from build123d import *

# Parameters (mm, degrees)
SKETCH_1_W          = 280
SKETCH_1_H          = 150
EXTRUDE_1_DEPTH     = 5
SKETCH_2_W          = 280
SKETCH_2_H          = 25
EXTRUDE_3_DEPTH     = 10
CUT_EXTRUDE_1_DEPTH = 500
SKETCH_7_R          = 4
CUT_EXTRUDE_2_DEPTH = 1000
SKETCH_8_W          = 112.049433073
SKETCH_8_H          = 25
CUT_EXTRUDE_3_DEPTH = 1000
SKETCH_9_W          = 5
SKETCH_9_H          = 160
EXTRUDE_4_DEPTH     = 20
EXTRUDE_5_DEPTH     = 5
CUT_EXTRUDE_4_DEPTH = 50
FILLET_1_R          = 2
FILLET_2_R          = 2


with BuildPart() as part:
    # 草图1 → 凸台-拉伸1 (new body)
    with BuildSketch(Plane.XY):
        Rectangle(SKETCH_1_W, SKETCH_1_H)
    extrude(amount=EXTRUDE_1_DEPTH)

    # 草图2 → 凸台-拉伸3 (add)
    with BuildSketch(Plane(origin=(0, 75, 0), x_dir=(1, 0, 0), z_dir=(0, 1, 0))):
        with Locations((0, -17.5)):
            Rectangle(SKETCH_2_W, SKETCH_2_H)
    extrude(amount=-EXTRUDE_3_DEPTH)

    # 草图6 → 切除-拉伸1 (cut, symmetric)
    with BuildSketch(Plane.XY.offset(5)):
        Polygon((154.593930268, -89.892698805), (-30, 65), (-77.119612047, 104.53804909), (-170.923908706, 102.008061066), (-172.604783039, -51.581831085), (-172.604783039, -108.521449105), align=None)
    extrude(amount=CUT_EXTRUDE_1_DEPTH, both=True, mode=Mode.SUBTRACT)

    # 草图7 → 切除-拉伸2 (cut)
    with BuildSketch(Plane.XZ.offset(-65)):
        with Locations(Location((-20, 20, 0), (0, 0, 270))):
            Circle(SKETCH_7_R)
        with Locations(Location((10, 20, 0), (0, 0, 270))):
            Circle(SKETCH_7_R)
    extrude(amount=-CUT_EXTRUDE_2_DEPTH, mode=Mode.SUBTRACT)

    # 草图8 → 切除-拉伸3 (cut)
    with BuildSketch(Plane.XZ.offset(-65)):
        with Locations((83.975283464, 17.5)):
            Rectangle(SKETCH_8_W, SKETCH_8_H)
    extrude(amount=-CUT_EXTRUDE_3_DEPTH, mode=Mode.SUBTRACT)

    # 草图9 → 凸台-拉伸4 (add)
    with BuildSketch(Plane(origin=(140, 0, 0), x_dir=(0, 0, -1), z_dir=(1, 0, 0))):
        with Locations((-2.5, -5)):
            Rectangle(SKETCH_9_W, SKETCH_9_H)
    extrude(amount=EXTRUDE_4_DEPTH)

    # 草图10 → 凸台-拉伸5 (add)
    with BuildSketch(Plane.XY.offset(5)):
        Polygon((136.845502963, -75), (140, -77.6469373), (140, -75), align=None)
    extrude(amount=-EXTRUDE_5_DEPTH)

    # 草图11 → 切除-拉伸4 (cut)
    with BuildSketch(Plane.XY.offset(5)):
        Polygon((140, -77.6469373), (159.760548741, -94.228006461), (119.027644691, -86.706463214), align=None)
    extrude(amount=-CUT_EXTRUDE_4_DEPTH, mode=Mode.SUBTRACT)

    # 圆角1
    fillet_1_edges = [part.edges().sort_by_distance(p)[0] for p in [
        (-1.024716536, 65, 5),
    ]]
    fillet(fillet_1_edges, radius=FILLET_1_R)

    # 圆角2
    fillet_2_edges = [part.edges().sort_by_distance(p)[0] for p in [
        (27.950566927, 69, 5),
    ]]
    fillet(fillet_2_edges, radius=FILLET_2_R)


solid = part.part
The model under review builds one solid part; all positions refer to its coordinate system, in mm. A direction names the side the tool comes from. Round coordinates to 2 decimals unless told otherwise and drop trailing zeros. Loops run counter-clockwise (first coordinate to the right, second up) from the corner with the lowest first, then second, coordinate; pieces in that order, holes last. Notation, with made-up numbers: M -35,85.25 L -27,85.25 A21 cw -27,105.25 Z; hole C 40.25,21.25 d10. An arc over 180 degrees is marked long. Answer as CSV lines item,"result".
1. Draft analysis for pull direction Z (two halves, no side actions). For faces 4 (the face through (10, 70, 24)), 5 (the face through (154, -85, 3)), 6 (the face through (80, 14, 0)), state which applies: pulls with the +Z half, pulls with the -Z half, needs draft (parallel to the pull), parting line crosses it, or undercut.
Outcome:
face 4,"undercut"
face 5,"needs draft"
face 6,"pulls with the -Z half"
2. We need section C-C (x = 10). Give the boundary of the cut face in (y, z), plus the area to 3 significant figures.
Outcome:
outline,"M 31.44,0 L 75,0 L 75,16 L 65,16 L 65,7 A2 cw 63,5 L 31.44,5 Z; M 65,24 L 75,24 L 75,30 L 65,30 Z"
area,"389 mm2"
3. Insertion check: pin 1 Ø8 at (x, z) = (39.5, 5) entering from -Y; pin 2 Ø4 at (x, y) = (96, -18.5) entering from +Z; pin 3 Ø6 at (x, z) = (45.5, 4) entering from -Y. Each pin has a flat end and moves straight along its axis. Give the tip position at first contact, or say it passes through.
Outcome:
pin 1,"stops at y = 3.33"
pin 2,"stops at z = 5"
pin 3,"stops at y = -0.87"
4. We need section D-D (y = 29). Give the boundary of the cut face in (x, z).
Outcome:
outline,"M 12.9,0 L 160,0 L 160,5 L 12.9,5 Z"
5. To check wall thickness, follow L1, parallel to X at y = 69, z = 20; L2, parallel to X at y = 68.25, z = 20; L3, parallel to Z at x = 78, y = 7. State the ranges of each line that lie inside material, in increasing order. Write a range as [from, to].
Outcome:
L1,"x = [-34.77, -24], [-16, 6], [14, 27.95]"
L2,"x = [-33.87, -24], [-16, 6], [14, 27.95]"
L3,"z = [0, 5]"
6. We need section A-A (z = 20). Give the boundary of the cut face in (x, y), plus the area to 3 significant figures.
Outcome:
outline,"M -41.92,75 L -30,65 L -24,65 L -24,75 Z; M -16,65 L 6,65 L 6,75 L -16,75 Z; M 14,65 L 27.95,65 L 27.95,75 L 14,75 Z"
area,"479 mm2"
7. For faces 1 (the face through (27.951, 70, 18)), 2 (the face through (-1, 65, 18)), 3 (the face through (160, -4, 3)), list the 3-axis set-ups (+Z, -Z, +X, -X, +Y, -Y) from which the entire face can be reached by the end or side of a thin tool; tool diameter is ignored.
Outcome:
face 1,"+Z, +X, +Y, -Y"
face 2,"+Z, +X, -X, -Y"
face 3,"+Z, -Z, +X, +Y, -Y"
8. We need section B-B (x = -20). Give the boundary of the cut face in (y, z).
Outcome:
outline,"M 56.61,0 L 75,0 L 75,16 L 65,16 L 65,7 A2 cw 63,5 L 56.61,5 Z; M 65,24 L 75,24 L 75,30 L 65,30 Z"
